Autodesk Inventor part; units mm, degrees
ref_plane "YZ Plane" through (0, 0, 0) normal (1, 0, 0) x (0, 1, 0)
ref_plane "XZ Plane" through (0, 0, 0) normal (0, 1, 0) x (-1, 0, 0)
ref_plane "XY Plane" through (0, 0, 0) normal (0, 0, 1) x (1, 0, 0)
sketch "Sketch1" plane through (0, 0, 0) normal (0, 1, 0) x (-1, 0, 0)
  line L0 (0, 0) -> (28, 0)
  line L1 (28, 0) -> (28, -38.5)
  line L2 (28, -38.5) -> (0, -38.5)
  line L3 (0, -38.5) -> (0, 0)
  line L4 (26, -6.25) -> (2, -6.25)
  line L5 (2, -6.25) -> (2, -32.25)
  line L6 (2, -32.25) -> (26, -32.25)
  line L7 (26, -32.25) -> (26, -6.25)
  dimension "d0" = 28
  dimension "d1" = 38.5
  dimension "d2" = 24
  dimension "d3" = 26
  dimension "d43" = 2
  dimension "d44" = 6.25
extrude "Extrusion1" add sketch "Sketch1" along normal blind 3
sketch "Sketch2" plane through (0, 3, 0) normal (0, 1, 0) x (1, 0, 0)
  line L0 (-28, 0) -> (0, 0)
  circle A0 centre (0, 0) radius 2
  circle A1 centre (-28, 0) radius 2
  line L1 (0, 38.5) -> (-28, 38.5)
  circle A2 centre (-28, 38.5) radius 2
  circle A3 centre (0, 38.5) radius 2
  dimension "d8" = 4
  dimension "d9" = 4
  dimension "d10" = 4
  dimension "d11" = 4
extrude "Extrusion2" cut sketch "Sketch2" against normal blind 3
sketch "Sketch3" plane through (0, 3, 0) normal (0, 1, 0) x (1, 0, 0)
  line L0 (-32.85, 43.35) -> (4.85, 43.35)
  line L1 (4.85, 43.35) -> (4.85, -4.85)
  line L2 (4.85, -4.85) -> (-32.85, -4.85)
  line L3 (-32.85, -4.85) -> (-32.85, 43.35)
  line L4 (-2, 38.5) -> (-26, 38.5)
  line L5 (0, 2) -> (0, 36.5)
  line L6 (-2, 32.25) -> (-2, 6.25)
  line L7 (-26, 6.25) -> (-26, 32.25)
  line L8 (-2, 6.25) -> (-26, 6.25)
  line L9 (-26, 6.25) -> (-26, 32.25)
  line L10 (-26, 32.25) -> (-2, 32.25)
  line L11 (-2, 32.25) -> (-2, 6.25)
  point P0 (0, 0)
  point P1 (-26, 6.25)
  dimension "d14" = 48.2
  dimension "d15" = 37.7
  dimension "d16" = 4.85
  dimension "d17" = 4.85
extrude "Extrusion3" add sketch "Sketch3" along normal blind 2
sketch "Sketch4" plane through (0, 3, 0) normal (0, -1, 0) x (1, 0, 0)
  circle A0 centre (2.35, -40.85) radius 2.25
  line L0 (-2, -38.5) -> (-26, -38.5)
  line L1 (0, -2) -> (0, -36.5)
  circle A1 centre (-30.35, -40.85) radius 2.25
  line L2 (-28, -36.5) -> (-28, -2)
  circle A2 centre (-30.35, 2.35) radius 2.25
  line L3 (-26, 0) -> (-2, 0)
  circle A3 centre (2.35, 2.35) radius 2.25
  point P0 (0, 0)
  dimension "d20" = 4.5
  dimension "d21" = 2.35
  dimension "d22" = 2.35
  dimension "d23" = 4.5
  dimension "d24" = 2.35
  dimension "d25" = 2.35
  dimension "d26" = 4.5
  dimension "d27" = 2.35
  dimension "d28" = 4.5
  dimension "d29" = 2.35
  dimension "d30" = 2.35
  dimension "d31" = 2.35
extrude "Extrusion4" add sketch "Sketch4" along normal blind 3
fillet "Fillet1" radius 2 4 edges at (4.85, 4, -43.35) (4.85, 4, 4.85) (-32.85, 4, 4.85) (-32.85, 4, -43.35)
sketch "Sketch5" plane through (0, 5, 0) normal (0, 1, 0) x (1, 0, 0)
  line L0 (-26, 32.25) -> (-2, 32.25)
  line L1 (-2, 6.25) -> (-26, 6.25)
  line L2 (-2, 32.25) -> (-2, 6.25)
  line L3 (-26, 6.25) -> (-26, 32.25)
  circle A0 centre (-2, 19.25) radius 1
  circle A1 centre (-29, 19.25) radius 1
  line L4 (4.85, -2.85) -> (4.85, 41.35)
  point P0 (0, 0)
  dimension "d45" = 2
  dimension "d46" = 2
  dimension "d47" = 13
  dimension "d50" = 13
  dimension "d73" = 27
  dimension "d75" = 3
extrude "Extrusion6" cut sketch "Sketch5" against normal through all contours A0 L2 | L2 A0 | A1
sketch "Sketch6" plane through (-28, 0, -36.5) normal (-1, 0, 0) x (0, 0, 1)
  line L0 (0, 0) -> (34.5, 0)
  line L1 (-4.85, 3) -> (39.35, 3)
  line L2 (20.25, 0) -> (14.25, 0)
  line L3 (14.25, 0) -> (14.25, 3)
  line L4 (14.25, 3) -> (20.25, 3)
  line L5 (20.25, 3) -> (20.25, 0)
  line L6 (41.35, 3) -> (41.35, 5)
  point P0 (36.5, 0)
  point P1 (41.35, 4)
  dimension "d53" = 6
  dimension "d54" = 21.1
extrude "Extrusion7" cut sketch "Sketch6" against normal blind 10
chamfer "Chamfer1" distance 2 angle 45 2 edges at (-27, 0, -22.25) (-27, 0, -16.25)
sketch "Sketch7" plane through (0, 5, 0) normal (0, 1, 0) x (1, 0, 0)
  line L0 (-30.85, -4.85) -> (2.85, -4.85)
  line L1 (-26, 6.25) -> (-26, 32.25)
  arc A0 (-26, 23.25) -> (-26, 15.25) centre (-19.0718, 19.25) ccw
  line L2 (-26, 23.25) -> (-26, 15.25)
  point P0 (0, 0)
  dimension "d63" = 8
  dimension "d64" = 20.1
  dimension "d65" = 8
extrude "Extrusion8" cut sketch "Sketch7" against normal blind 10
sketch "Sketch8" plane through (0, 5, 0) normal (0, 1, 0) x (1, 0, 0)
  circle A0 centre (-14, 3.125) radius 1.75
  line L0 (-2, 6.25) -> (-26, 6.25)
  line L1 (-26, 0) -> (-2, 0)
  line L2 (-32.85, 41.35) -> (-32.85, -2.85)
  point P0 (0, 0)
  dimension "d68" = 3.5
  dimension "d69" = 3.125
  dimension "d70" = 18.85
extrude "Extrusion9" cut sketch "Sketch8" against normal through all
sketch "Sketch9" plane through (0, 5, 0) normal (0, 1, 0) x (1, 0, 0)
  circle A0 centre (-14, 3.125) radius 1.75
  line L0 (-15, 4.5611) -> (-15, 6.25)
  line L1 (-15, 6.25) -> (-13, 6.25)
  line L2 (-13, 6.25) -> (-13, 4.5611)
  arc A1 (-13, 4.5611) -> (-15, 4.5611) centre (-14, 3.125) ccw
  line L3 (-2, 6.25) -> (-26, 6.25)
  point P0 (0, 0)
  point P1 (-14, 6.25)
  dimension "d76" = 2
  dimension "d77" = 1
extrude "Extrusion10" cut sketch "Sketch9" against normal through all contours A0 L0 L1 L2
fillet "Fillet2" radius 2 2 edges at (-15, 2.5, -4.5611) (-13, 2.5, -4.5611)
properties part number "ServoFullMountInsert"
Build history of the part. All positions in model axes, mm. A direction names the side the tool comes from. Give positions to 0.01 mm unless a question says otherwise; leave off trailing zeros. Loops run counter-clockwise (first coordinate to the right, second up) from the corner with the lowest first, then second, coordinate; pieces in that order, holes last.
Item 1: Slice it at D-D, the plane x = 1. List the corners of the cut face in (y, z), and give its area (3 significant figures).
Answers follow:
outline: (0, -42.65) - (3, -42.65) - (3, -43.35) - (5, -43.35) - (5, 4.85) - (3, 4.85) - (3, 4.15) - (0, 4.15) - (0, 0.55) - (3, 0.55) - (3, -39.05) - (0, -39.05) - close
area: 118 mm2
Item 2: Slice it at C-C, the plane z = -35. List the corners of the cut face in (x, y).
Answers follow:
outline: (-32.85, 3) - (-28, 3) - (-28, 0) - (0, 0) - (0, 3) - (4.85, 3) - (4.85, 5) - (-32.85, 5) - close
Item 3: Flat gauge pins, fed straight in: pin 1 (1.5 mm diameter, centred on y = 1.5, z = -26.5, fed in from -X); pin 2 (1.5 mm diameter, centred on y = 2, z = -28.5, fed in from +X); pin 3 (2.5 mm diameter, centred on x = -11, y = 1.5, fed in from +Z); pin 4 (4 mm diameter, centred on x = -23, z = -18, fed in from -Y). Where does each tip first touch, or does it go through?
Answers follow:
pin 1: stops at x = -28
pin 2: stops at x = 0
pin 3: stops at z = 0
pin 4: passes through
Item 4: Which spindle directions (+Z, -Z, +X, -X, +Y, -Y) get a long thin tool onto all of the face, cutting with end or side? Do faces 1 (the face through (-14, 1, 0)), 2 (the face through (-28.204, 1.521, -41.526)), 3 (the face through (-27.3, 2.5, -16.25)), 4 (the face through (-7, 2, -6.25)). Say none if no direction does.
Answers follow:
face 1: +Z, +X, -X, -Y
face 2: -Y
face 3: -X, -Y
face 4: +Y, -Y
Item 5: Slice it at A-A, the plane x = -29. List the corners of the cut face in (y, z), and give its area (3 significant figures).
Answers follow:
outline: (0, -42.65) - (3, -42.65) - (3, -43.35) - (5, -43.35) - (5, -20.25) - (3, -20.25) - (3, -39.05) - (0, -39.05) - close; (0, 0.55) - (3, 0.55) - (3, -18.25) - (5, -18.25) - (5, 4.85) - (3, 4.85) - (3, 4.15) - (0, 4.15) - close
area: 114 mm2
Item 6: Pull direction X, two halves, no side cores. Call faces 5 (the face through (-1.7, 5, -24.9)), 6 (the face through (-32.28, 4.01, 4.25)), 7 (the face through (-2, 2, -26)): released by +X, released by -X, zero draft, split by the parting line, or undercut.
Answers follow:
face 5: zero draft
face 6: released by -X
face 7: undercut
Item 7: Drill centre lines: line 1 (X direction, y = 4.4, z = -19.25); line 2 (Z direction, x = -7, y = 0.95); line 3 (Z direction, x = -14, y = 1) (3 decimals). Where is each one in solid material? Low to high.
Answers follow:
line 1: x = -32.85 to -30, -28 to -27.07, -1 to 4.85
line 2: z = -38.5 to -32.25, -6.25 to 0
line 3: z = -38.5 to -32.25, -1.375 to 0
Item 8: Slice it at B-B, the plane z = -27. List the corners of the cut face in (x, y), and give its area (3 significant figures).
Answers follow:
outline: (-32.85, 3) - (-28, 3) - (-28, 0) - (-26, 0) - (-26, 5) - (-32.85, 5) - close; (-2, 0) - (0, 0) - (0, 3) - (4.85, 3) - (4.85, 5) - (-2, 5) - close
area: 39.4 mm2
